Could you check a few things on this model? Use its own coordinates, in mm. A direction names the side the tool comes from. Give positions to 0.01 mm unless a question says otherwise; leave off trailing zeros. Loops run counter-clockwise (first coordinate to the right, second up) from the corner with the lowest first, then second, coordinate; pieces in that order, holes last.
1. For faces 1 (the flat face through (-5, 2, 0)), 2 (the cylindrical face through (-1.08, -4.88, -9.83)), which set-ups out of +Z, -Z, +X, -X, +Y, -Y let a thin tool reach every point of the face, with its end or its side?
2. Imagine slicing it at C-C (z = 15.5). List the corners of the cut face in (x, y) for me, plus the area to 3 significant figures.
3. For P1, Ø6, axis at y = -4, z = 9, coming from the -X side; P2, Ø9, axis at x = 0, y = 0, coming from the -Z side; P3, Ø3, axis at y = 4, z = 2.5, coming from the -X side; P4, Ø5, axis at x = 4, z = -12, coming from the -Y side, each with a flat end and sliding along its axis, tell me the tip position at first contact or that it passes through.
4. I need wall thicknesses on line 1 along Y through (x, z) = (0, -6); line 2 along Y through (x, z) = (0, 8.75); line 3 along X through (y, z) = (1.75, -14.5). Which ranges of each line are inside material? Lowest first, please.
5. Thinking about a two-plate mould opening in X: for faces 3 (the flat face through (6, 0, -19.939)), 4 (the cylindrical face through (-1.95, -14.86, -0.27)), 5 (the cylindrical face through (6.687, 2.106, 10.109)), which applies, +X half, -X half, draft (parallel to the pull), parting line (faces both ways), or undercut?
6. Imagine slicing it at D-D (z = -8.5). List the corners of the cut face in (x, y) for me.
7. Imagine slicing it at A-A (x = 0). List the corners of the cut face in (y, z) for me, plus the area to 3 significant figures.
Autodesk Inventor part; units mm, degrees
ref_plane "YZ Plane" through (0, 0, 0) normal (1, 0, 0) x (0, 1, 0)
ref_plane "XZ Plane" through (0, 0, 0) normal (0, 1, 0) x (-1, 0, 0)
ref_plane "XY Plane" through (0, 0, 0) normal (0, 0, 1) x (1, 0, 0)
sketch "Sketch12" plane through (0, 0, 0) normal (0, 0, 1) x (1, 0, 0)
  circle A0 centre (0, 0) radius 14.986
  circle A1 centre (0, 0) radius 5
  dimension "d107" = 29.972
  dimension "d108" = 10
extrude "Extrusion1" add sketch "Sketch12" along normal mid plane 39.878
sketch "Sketch13" plane through (0, 0, 19.939) normal (0, 0, 1) x (1, 0, 0)
  circle A0 centre (0, 0) radius 5 construction
  circle A1 centre (0, 0) radius 7.0104
  dimension "d111" = 14.0208
extrude "Extrusion2" cut sketch "Sketch13" against normal blind 19.939
fillet "Fillet1" radius 0.762 2 edges at (-14.986, 0, -19.939) (-14.986, 0, 19.939)
equation "\"BendRadius\" = Thickness"
equation "\"BendReliefWidth\" = Thickness"
equation "\"BendReliefDepth\" = 0.5 * Thickness"
equation "\"CornerReliefSize\" = 4 * Thickness"
equation "\"MinimumRemnant\" = 2 * Thickness"
equation "\"TransitionRadius\" = BendRadius"
equation "\"JacobiRadiusSize\" = BendRadius"
equation "\"GapSize\" = Thickness"
properties part number "Shaft Coupler" material "Steel, Mild"
Derived:
1. face 1: +Z
1. face 2: +Z, -Z
2. outline: circle Ø29.97 at (0, 0); hole circle Ø14.02 at (0, 0)
2. area: 551 mm2
3. P1: stops at x = -14.95
3. P2: passes through
3. P3: stops at x = -14.78
3. P4: stops at y = -14.91
4. line 1: y = -14.99 to -5, 5 to 14.99
4. line 2: y = -14.99 to -7.01, 7.01 to 14.99
4. line 3: x = -14.88 to -4.68, 4.68 to 14.88
5. face 3: draft
5. face 4: parting line
5. face 5: undercut
6. outline: circle Ø29.97 at (0, 0); hole circle Ø10 at (0, 0)
7. outline: (-14.99, -19.18) arc R0.76 ccw to (-14.22, -19.94) - (-5, -19.94) - (-5, 0) - (-7.01, 0) - (-7.01, 19.94) - (-14.22, 19.94) arc R0.76 ccw to (-14.99, 19.18) - close; (5, -19.94) - (14.22, -19.94) arc R0.76 ccw to (14.99, -19.18) - (14.99, 19.18) arc R0.76 ccw to (14.22, 19.94) - (7.01, 19.94) - (7.01, 0) - (5, 0) - close
7. area: 716 mm2
